from build123d import *

# Parameters (mm, degrees)
SKETCH_1_R      = 3.9
SKETCH_1_R_2    = 2.6
EXTRUDE_1_DEPTH = 15
EXTRUDE_START   = -7
SKETCH_2_R      = 2.6
EXTRUDE_2_DEPTH = 7
EXTRUDE_START_2 = 6.2
EXTRUDE_3_DEPTH = 6.2
CHAMFER_1_SIZE  = 0.3
CHAMFER_2_SIZE  = 0.3
CHAMFER_3_SIZE  = 0.3


with BuildPart() as part:
    # 草图1 → 凸台-拉伸1 (new body)
    with BuildSketch(Plane.XY):
        Circle(SKETCH_1_R)
        Circle(SKETCH_1_R_2, mode=Mode.SUBTRACT)
    extrude(amount=EXTRUDE_1_DEPTH)

    # 草图2 → 凸台-拉伸2 (add)
    with BuildSketch(Plane.XY.offset(15).offset(EXTRUDE_START)):
        Circle(SKETCH_2_R)
    extrude(amount=EXTRUDE_2_DEPTH)

    # 草图3 → 凸台-拉伸3 (add)
    with BuildSketch(Plane(origin=(0, 0, 8), x_dir=(-1, 0, 0), z_dir=(0, 0, -1)).offset(EXTRUDE_START_2)):
        with BuildLine():
            Line((-1.6, -2.049390153), (-1.6, 2.049390153))
            ThreePointArc((-1.6, 2.049390153), (-2.6, 0), (-1.6, -2.049390153))
        make_face()
        with BuildLine():
            ThreePointArc((2.6, 0), (2.336664289, 1.140175425), (1.6, 2.049390153))
            Line((1.6, 2.049390153), (1.6, -2.049390153))
            ThreePointArc((1.6, -2.049390153), (2.336664289, -1.140175425), (2.6, 0))
        make_face()
    extrude(amount=-EXTRUDE_3_DEPTH)

    # 倒角1
    chamfer_1_edges = [part.edges().sort_by_distance(p)[0] for p in [
        (-2.6, 0, 0),
    ]]
    chamfer(chamfer_1_edges, length=CHAMFER_1_SIZE)

    # 倒角2
    chamfer_2_edges = [part.edges().sort_by_distance(p)[0] for p in [
        (-3.9, 0, 0),
    ]]
    chamfer(chamfer_2_edges, length=CHAMFER_2_SIZE)

    # 倒角3
    chamfer_3_edges = [part.edges().sort_by_distance(p)[0] for p in [
        (1.6, 0, 1.8),
        (-1.6, 0, 1.8),
    ]]
    chamfer(chamfer_3_edges, length=CHAMFER_3_SIZE)


solid = part.part
Build history of the part. All positions in model axes, mm. Coordinates: 2 decimals unless noted, no trailing zeros. Order: outer loops, then holes, each group sorted by start corner. A loop starts at its lowest first (then second) coordinate and runs counter-clockwise, first axis right, second up. Notation, with made-up numbers: (43, -7) -> (55, -7) arc R8 ccw to (55, 1) -> close; hole circle Ø9 at (21, 30.5). An arc over 180 degrees is marked (long way). One line per item, written item: value.
(1) Slice it at C-C, the plane x = 0. List the corners of the cut face in (y, z), plus the area to 3 significant figures.
Checked values:
outline: (-3.9, 0.3) -> (-3.6, 0) -> (-2.9, 0) -> (-2.6, 0.3) -> (-2.6, 8) -> (2.6, 8) -> (2.6, 0.3) -> (2.9, 0) -> (3.6, 0) -> (3.9, 0.3) -> (3.9, 15) -> (-3.9, 15) -> close
area: 75.2 mm2
(2) Probe line 1 (Y direction, x = 0, z = 3.25); line 2 (X direction, y = 0.25, z = 3.75); line 3 (Y direction, x = -1.5, z = 5). List the from-to ranges inside material, lowest first. Write a range as [from, to].
Checked values:
line 1: [-3.9, -2.6], [2.6, 3.9]
line 2: [-3.89, -1.6], [1.6, 3.89]
line 3: [-3.6, -2.12], [2.12, 3.6]
(3) Slice it at A-A, the plane y = 0. List the corners of the cut face in (x, z), plus the area to 3 significant figures.
Checked values:
outline: (-3.9, 0.3) -> (-3.6, 0) -> (-2.9, 0) -> (-2.6, 0.3) -> (-2.6, 1.8) -> (-1.9, 1.8) -> (-1.6, 2.1) -> (-1.6, 8) -> (1.6, 8) -> (1.6, 2.1) -> (1.9, 1.8) -> (2.6, 1.8) -> (2.6, 0.3) -> (2.9, 0) -> (3.6, 0) -> (3.9, 0.3) -> (3.9, 15) -> (-3.9, 15) -> close
area: 87.5 mm2
(4) Mould opens along Y. For faces 1 (the flat face through (0, 0, 15)), 2 (the cylindrical face through (-2.87, 2.64, 7.55)), 3 (the flat face through (1.6, 0, 5)), 4 (the flat face through (-1.6, 0, 5)) say: pulls with the +Y half, pulls with the -Y half, needs draft (parallel to the pull), parting line crosses it, or undercut.
Checked values:
face 1: needs draft
face 2: parting line crosses it
face 3: undercut
face 4: undercut
(5) Slice it at B-B, the plane z = 3.5. List the corners of the cut face in (x, y), plus the area to 3 significant figures.
Checked values:
outline: circle Ø7.8 at (0, 0); hole (-1.6, -2.05) arc R2.6 ccw to (1.6, -2.05) -> (1.6, 2.05) arc R2.6 ccw to (-1.6, 2.05) -> close
area: 32.3 mm2
(6) Slice it at D-D, the plane z = 8.5. List the corners of the cut face in (x, y), plus the area to 3 significant figures.
Checked values:
outline: circle Ø7.8 at (0, 0)
area: 47.8 mm2
(7) Drop flat-ended pins along their axis: pin 1 Ø1 at (y, z) = (2, 9) entering from -X; pin 2 Ø0.6 at (x, y) = (-2, -1) entering from -Z; pin 3 Ø2.5 at (x, y) = (-0.5, 1) entering from -Z. Give the stop position or say it passes through.
Checked values:
pin 1: x = -3.6
pin 2: z = 1.8
pin 3: z = 1.95
